Can you work these out from the drawing? Everything is in mm from the part's minimum corner. A direction names the side the tool comes from. Round coordinates to 2 decimals unless told otherwise and drop trailing zeros. Write each loop counter-clockwise with the first axis right and the second up, starting at its lowest first coordinate (ties: lowest second). Pieces come first, ordered by that corner, then holes.
Q1. Please list where these lines run through material, in increasing order: line 1 along X through (y, z) = (41, 64.5) (3 decimals); line 2 along Y through (x, z) = (71.5, 38.1) (1 decimal); line 3 along Y through (x, z) = (101, 9.5).
Q2. If we section it at B-B (y = 151): Please give me the cut outline in (x, z) (3 decimals).
Q3. If we section it at C-C (x = 42): Please give me the cut outline in (y, z) (3 decimals), plus the area to 3 significant figures.
Q4. If we section it at D-D (z = 11): Please give me the cut outline in (x, y) (1 decimal), plus the area to 3 significant figures.
Q5. If we section it at A-A (z = 38.1): Please give me the cut outline in (x, y) (1 decimal), plus the area to 3 significant figures.
Q6. For the marked faces 4, 5 and 6, which set-ups out of +Z, -Z, +X, -X, +Y, -Y let a thin tool reach every point of the face, with its end or its side?
Q7. We'd pull the mould along X, two halves only. Please class the marked faces 1, 2 and 3: +X half, -X half, draft (parallel to the pull), parting line (faces both ways), or undercut.
Q8. I'm going to push flat-ended pins straight in: pin 1 Ø4 at (x, z) = (50.5, 23.5) entering from +Y (3 decimals); pin 2 Ø1 at (y, z) = (106.5, 55.5) entering from +X; pin 3 Ø15 at (x, z) = (91.5, 69.5) entering from +Y. Where does each tip first touch, or does it pass through?
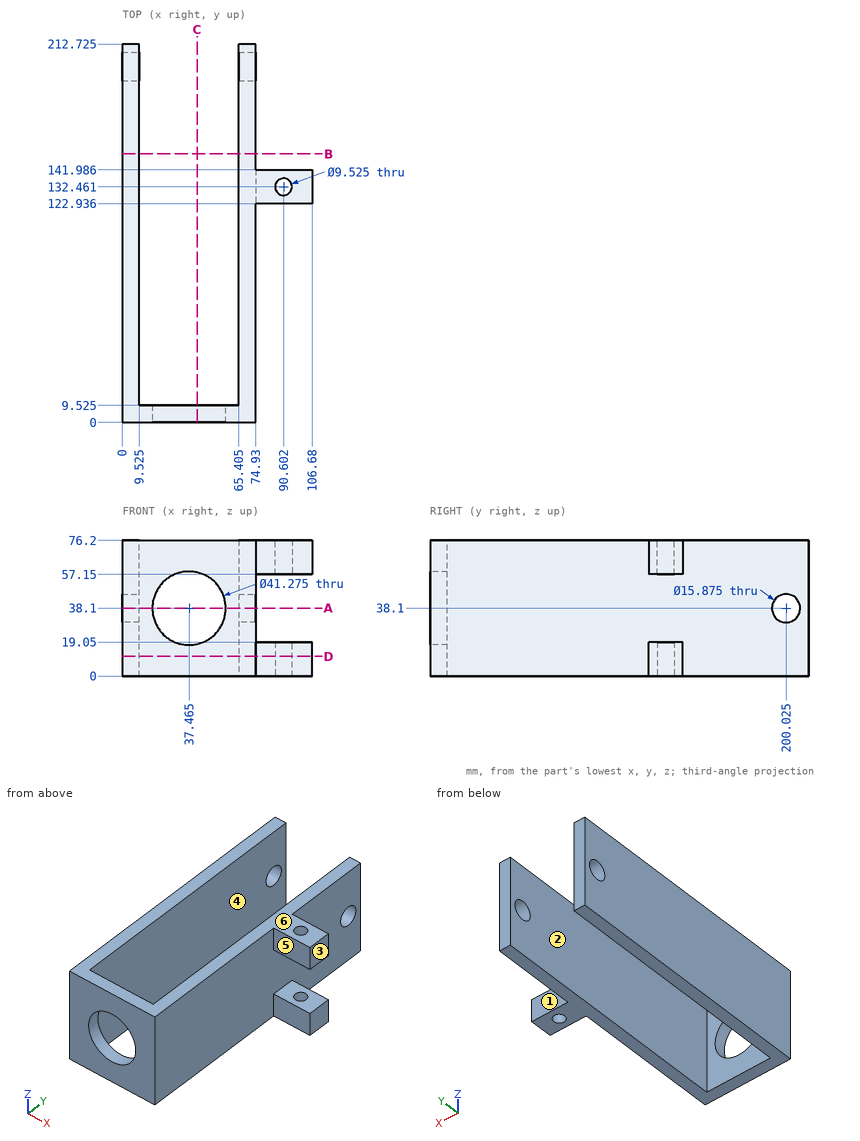
A:
1. line 1: x = 0 to 9.525, 65.405 to 74.93
1. line 2: y = 0 to 192.1, 208 to 212.7
1. line 3: y = 122.94 to 141.99
2. outline: (0, 0) - (9.525, 0) - (9.525, 76.2) - (0, 76.2) - close; (65.405, 0) - (74.93, 0) - (74.93, 76.2) - (65.405, 76.2) - close
3. outline: (0, 0) - (9.525, 0) - (9.525, 17.967) - (0, 17.967) - close; (0, 58.233) - (9.525, 58.233) - (9.525, 76.2) - (0, 76.2) - close
3. area: 342 mm2
4. outline: (0, 0) - (74.9, 0) - (74.9, 122.9) - (106.7, 122.9) - (106.7, 142) - (74.9, 142) - (74.9, 212.7) - (65.4, 212.7) - (65.4, 9.5) - (9.5, 9.5) - (9.5, 212.7) - (0, 212.7) - close; hole circle Ø9.5 at (90.6, 132.5)
4. area: 5,120 mm2
5. outline: (0, 0) - (16.8, 0) - (16.8, 9.5) - (9.5, 9.5) - (9.5, 192.1) - (0, 192.1) - close; (0, 208) - (9.5, 208) - (9.5, 212.7) - (0, 212.7) - close; (58.1, 0) - (74.9, 0) - (74.9, 192.1) - (65.4, 192.1) - (65.4, 9.5) - (58.1, 9.5) - close; (65.4, 208) - (74.9, 208) - (74.9, 212.7) - (65.4, 212.7) - close
5. area: 3,890 mm2
6. face 4: +Z, -Z, +Y
6. face 5: +Z, -Z, +X, -Y
6. face 6: +Z, +X, -X, +Y, -Y
7. face 1: draft
7. face 2: undercut
7. face 3: +X half
8. pin 1: stops at y = 9.525
8. pin 2: stops at x = 74.93
8. pin 3: stops at y = 141.99
